```python
from build123d import *

# Parameters (mm, degrees)
F2_R = 9
F3_R = 9
F4_R = 8
F5_R = 0.5


with BuildPart() as f1:
    # F0 (on Front) → F1 (revolve)
    with BuildSketch(Plane.XZ):
        Polygon((0, 4.5), (0, 0), (64, 0), (64, 9.5), (24, 9.5), (8.380214, 4.5), align=None)
    revolve(axis=Axis((32, 0, 0), (1, 0, 0)))

    # F2
    f2_edges = [f1.edges().sort_by_distance(p)[0] for p in [
        (64, 0, -9.5),
    ]]
    fillet(f2_edges, radius=F2_R)

    # F3
    f3_edges = [f1.edges().sort_by_distance(p)[0] for p in [
        (24, 0, -9.5),
    ]]
    fillet(f3_edges, radius=F3_R)

    # F4
    f4_edges = [f1.edges().sort_by_distance(p)[0] for p in [
        (8.380214, 0, -4.5),
    ]]
    fillet(f4_edges, radius=F4_R)

    # F5
    f5_edges = [f1.edges().sort_by_distance(p)[0] for p in [
        (0, 0, -4.5),
    ]]
    fillet(f5_edges, radius=F5_R)


solid = f1.part
```
The model under review builds one solid part; all positions refer to its coordinate system, in mm. A direction names the side the tool comes from. Round coordinates to 2 decimals unless told otherwise and drop trailing zeros. Loops run counter-clockwise (first coordinate to the right, second up) from the corner with the lowest first, then second, coordinate; pieces in that order, holes last. Notation, with made-up numbers: (18, 45.25) -> (64, 45.25) arc R27 cw to (64, 81.25) -> close; hole circle Ø2 at (42, -3). An arc over 180 degrees is marked (long way). Answer in a Markdown table with one row per item.
1) For pin 1 Ø3 at (x, y) = (34.5, -5.5) entering from +Z; pin 2 Ø3 at (x, y) = (31.5, 0.5) entering from -Z; pin 3 Ø3 at (x, z) = (9.5, -5.5) entering from +Y; pin 4 Ø8 at (x, y) = (19.5, -5.5) entering from -Z, all flat-tipped, find the tip position at first contact; note any pin that passes through.
Taken from the geometry:
| item | result |
|---|---|
| pin 1 | stops at z = 8.62 |
| pin 2 | stops at z = -9.5 |
| pin 3 | stops at y = 2.92 |
| pin 4 | stops at z = -8.56 |
2) Wall thickness on line 1 along Z through (x, y) = (47, 0.5); line 2 along Z through (x, y) = (56, -1.5); line 3 along Y through (x, z) = (13.5, 4.5): over which ranges is each line inside the solid? List them lowest first.
Taken from the geometry:
| item | result |
|---|---|
| line 1 | z = -9.49 to 9.49 |
| line 2 | z = -9.32 to 9.32 |
| line 3 | y = -4.18 to 4.18 |
3) Tool access review of faces 1 (the cylindrical face through (3.769, -1.352, 4.292)), 2 (the cylindrical face through (40, -9.42, -1.24)): name each direction out of +Z, -Z, +X, -X, +Y, -Y from which nothing blocks a thin tool from reaching the whole face with its end or side.
Taken from the geometry:
| item | result |
|---|---|
| face 1 | -X |
| face 2 | +X, -X |
4) Consider section A-A, the plane x = 43.5. Write out the cut boundary in (y, z), plus the area to 3 significant figures.
Taken from the geometry:
| item | result |
|---|---|
| outline | circle Ø19 at (0, 0) |
| area | 284 mm² |
